from build123d import *

# Parameters (mm, degrees)
F0_R     = 3.175
F1_DEPTH = 3.048


with BuildPart() as f1:
    # F0 (on Front) → F1 (new body)
    with BuildSketch(Plane.XZ):
        with BuildLine():
            ThreePointArc((-15.750488, 65.484375), (0, 79.375), (15.750488, 65.484375))
            Line((15.750488, 65.484375), (9.525, 114.3))
            ThreePointArc((9.525, 114.3), (-0.596483, 104.793695), (-9.450293, 115.490625))
            Line((-9.450293, 115.490625), (-15.750488, 65.484375))
        make_face()
        with Locations((-1.5875, 99.990685)):
            Circle(F0_R, mode=Mode.SUBTRACT)
        with BuildLine():
            ThreePointArc((15.750488, 61.515625), (15.843841, 62.505861), (15.875, 63.5))
            ThreePointArc((15.875, 63.5), (15.843841, 64.494139), (15.750488, 65.484375))
            ThreePointArc((15.750488, 65.484375), (0, 79.375), (-15.750488, 65.484375))
            ThreePointArc((-15.750488, 65.484375), (-15.843841, 64.494139), (-15.875, 63.5))
            Line((-15.875, 63.5), (-15.560644, 60.356436))
            ThreePointArc((-15.560644, 60.356436), (0.587316, 47.635868), (15.750488, 61.515625))
        make_face()
        with Locations((0, 63.5)):
            Circle(F0_R, mode=Mode.SUBTRACT)
        with BuildLine():
            Line((10.127114, 16.881475), (15.750488, 61.515625))
            ThreePointArc((15.750488, 61.515625), (0.587316, 47.635868), (-15.560644, 60.356436))
            Line((-15.560644, 60.356436), (-9.525, 0))
            ThreePointArc((-9.525, 0), (0, 9.525), (9.525, 0))
            ThreePointArc((9.525, 0), (6.970557, -6.491299), (0.677344, -9.500886))
            Line((0.677344, -9.500886), (44.732405, -7.932475))
            ThreePointArc((44.732405, -7.932475), (36.513756, -0.141225), (44.45, 7.9375))
            Line((44.45, 7.9375), (18.014958, 7.9375))
            ThreePointArc((18.014958, 7.9375), (12.052308, 10.629137), (10.127114, 16.881475))
        make_face()
        with BuildLine():
            ThreePointArc((-9.450293, 115.490625), (-0.596483, 104.793695), (9.525, 114.3))
            ThreePointArc((9.525, 114.3), (0.596483, 123.806305), (-9.450293, 115.490625))
        make_face()
        with Locations((0, 114.3)):
            Circle(F0_R, mode=Mode.SUBTRACT)
        with BuildLine():
            ThreePointArc((-15.875, 63.5), (-15.796215, 61.920378), (-15.560644, 60.356436))
            Line((-15.560644, 60.356436), (-15.875, 63.5))
        make_face()
        with BuildLine():
            ThreePointArc((9.525, 0), (0, 9.525), (-9.525, 0))
            ThreePointArc((-9.525, 0), (-6.735192, -6.735192), (0, -9.525))
            Line((0, -9.525), (0.677344, -9.500886))
            ThreePointArc((0.677344, -9.500886), (6.970557, -6.491299), (9.525, 0))
        make_face()
        Circle(F0_R, mode=Mode.SUBTRACT)
        with BuildLine():
            Line((0.677344, -9.500886), (0, -9.525))
            ThreePointArc((0, -9.525), (0.338886, -9.51897), (0.677344, -9.500886))
        make_face()
        with BuildLine():
            ThreePointArc((52.3875, 0), (50.06266, 5.61266), (44.45, 7.9375))
            ThreePointArc((44.45, 7.9375), (36.513756, -0.141225), (44.732405, -7.932475))
            ThreePointArc((44.732405, -7.932475), (50.161633, -5.51191), (52.3875, 0))
        make_face()
        with Locations((44.45, 0)):
            Circle(F0_R, mode=Mode.SUBTRACT)
    extrude(amount=F1_DEPTH)


solid = f1.part
The model under review builds one solid part; all positions refer to its coordinate system, in mm. A direction names the side the tool comes from. Give positions to 0.01 mm unless a question says otherwise; leave off trailing zeros. Order: outer loops, then holes, each group sorted by start corner. A loop starts at its lowest first (then second) coordinate and runs counter-clockwise, first axis right, second up. Notation, with made-up numbers: M 64,50 L 115,50 A17 cw 115,59 Z; hole C 76.25,23.25 d2. An arc over 180 degrees is marked long. Use one line per item in the form item = value. Start each with the question number.
Item 1: We need section C-C on z = 52. Give the boundary of the cut face in (x, y) (3 decimals).
Item 2: We need section A-A on x = -1.5. Give the boundary of the cut face in (y, z), plus the area to 3 significant figures.
Item 3: Insertion check: pin 1 Ø10 at (x, z) = (44.45, 0) entering from +Y; pin 2 Ø1.5 at (y, z) = (-2, 23) entering from -X; pin 3 Ø1.5 at (x, y) = (32.5, -1) entering from +Z. Each pin has a flat end and moves straight along its axis. Give the tip position at first contact, or say it passes through.
Item 4: We need section B-B on y = -1.35. Give the number of separate pieces and of enclosed holes in the cut face, plus the area to 3 significant figures.
Item 5: We need section D-D on x = 39.5. Give the boundary of the cut face in (y, z).
Item 6: For faces 4 (the flat face through (31, -2, 7.938)), 5 (the flat face through (12.9, -1.5, 38.9)), 6 (the cylindrical face through (-0.69, -1.5, 111.2)), list the 3-axis set-ups (+Z, -Z, +X, -X, +Y, -Y) from which the entire face can be reached by the end or side of a thin tool; tool diameter is ignored.
Item 7: The part is to be moulded in two halves that separate along Z. For faces 1 (the cylindrical face through (1.707, -1.503, 66.177)), 2 (the flat face through (3, 0, 43)), 3 (the flat face through (-12.556, -1.503, 90.838)), say which applies: pulls with the +Z half, pulls with the -Z half, needs draft (parallel to the pull), parting line crosses it, or undercut.
Item 8: To check wall thickness, follow line 1 along Z through (x, y) = (44.45, -1.3) (1 decimal); line 2 along X through (y, z) = (-2.1, 61); line 3 along Z through (x, y) = (44, -1.8). State the ranges of each line that lie inside material, in increasing order. Write a range as from..to.
Completed:
q1.outline = M -14.725,-3.048 L 14.552,-3.048 L 14.552,0 L -14.725,0 Z
q2.outline = M -3.05,-9.41 L 0,-9.41 L 0,-2.8 L -3.05,-2.8 Z; M -3.05,2.8 L 0,2.8 L 0,60.7 L -3.05,60.7 Z; M -3.05,66.3 L 0,66.3 L 0,96.82 L -3.05,96.82 Z; M -3.05,103.16 L 0,103.16 L 0,111.5 L -3.05,111.5 Z; M -3.05,117.1 L 0,117.1 L 0,123.71 L -3.05,123.71 Z
q2.area = 335 mm²
q3.pin_1 = 0
q3.pin_2 = -11.9
q3.pin_3 = 7.94
q4.separate_pieces = 1
q4.enclosed_holes = 5
q4.area = 3,710 mm²
q5.outline = M -3.05,-8.12 L 0,-8.12 L 0,7.94 L -3.05,7.94 Z
q6.face_4 = +Z, +X, +Y, -Y
q6.face_5 = +X, +Y, -Y
q6.face_6 = +Y, -Y
q7.face_1 = undercut
q7.face_2 = needs draft
q7.face_3 = pulls with the +Z half
q8.line_1 = -7.9..-3.2, 3.2..7.9
q8.line_2 = -15.68..-1.96, 1.96..15.69
q8.line_3 = -7.96..-3.14, 3.14..7.94
